```python
from build123d import *

# Parameters (mm, degrees)
SALIENTE_EXTRUIR1_DEPTH = 5
CORTAR_EXTRUIR1_DEPTH   = 15
SALIENTE_EXTRUIR2_DEPTH = 20
CORTAR_EXTRUIR2_DEPTH   = 30


with BuildPart() as part:
    # Croquis1 → Saliente-Extruir1 (new, symmetric)
    with BuildSketch(Plane.XY):
        Polygon((-2.5, 4), (2.5, -1), (-22.5, -8), (-22.5, -4), align=None)
        Polygon((22.5, 4), (-2.5, 4), (2.5, -1), (22.5, -1), align=None)
    extrude(amount=SALIENTE_EXTRUIR1_DEPTH, both=True)

    # Croquis3 → Cortar-Extruir1 (cut, symmetric)
    with BuildSketch(Plane(origin=(0, 0, 0), x_dir=(1, 0, 0), z_dir=(0, 1, 0))):
        Polygon((-22.5, 1.5), (-2.5, 5), (-22.5, 5), align=None)
        Polygon((-2.5, -5), (-22.5, -5), (-22.5, -1.5), align=None)
    extrude(amount=CORTAR_EXTRUIR1_DEPTH, both=True, mode=Mode.SUBTRACT)

    # Croquis5 → Saliente-Extruir2 (add)
    with BuildSketch(Plane.XY.offset(5)):
        Polygon((-2.5, 4), (-2.5, -2.4), (2.5, -1), (22.5, -1), (22.5, 4), align=None)
    extrude(amount=SALIENTE_EXTRUIR2_DEPTH)

    # Croquis2 → Cortar-Extruir2 (cut)
    with BuildSketch(Plane(origin=(0, 4, 0), x_dir=(1, 0, 0), z_dir=(0, 1, 0))):
        with BuildLine():
            Line((7.25, 0), (7.25, -20))
            ThreePointArc((7.25, -20), (6, -21.25), (4.75, -20))
            Line((4.75, -20), (4.75, 0))
            ThreePointArc((4.75, 0), (6, 1.25), (7.25, 0))
        make_face()
        with BuildLine():
            Line((15.25, 0), (15.25, -20))
            ThreePointArc((15.25, -20), (16.5, -21.25), (17.75, -20))
            Line((17.75, -20), (17.75, 0))
            ThreePointArc((17.75, 0), (16.5, 1.25), (15.25, 0))
        make_face()
    extrude(amount=-CORTAR_EXTRUIR2_DEPTH, mode=Mode.SUBTRACT)


solid = part.part
```
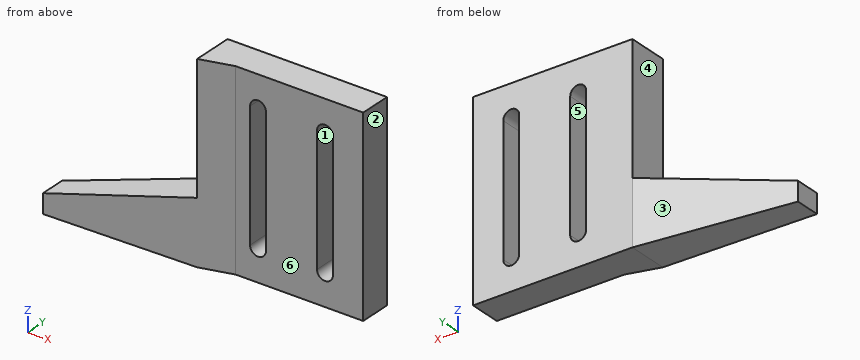
The listing builds one solid part. Answer for the finished solid, in the listing's coordinates (mm). Face numbers are marked on the shaded views. A direction names the side the tool comes from. Round coordinates to 2 decimals unless told otherwise and drop trailing zeros. Loops run counter-clockwise (first coordinate to the right, second up) from the corner with the lowest first, then second, coordinate; pieces in that order, holes last. Notation, with made-up numbers: (-20, 15) - (19, 15) arc R7 cw to (19, 28) - close; hole circle Ø2 at (53, 76.5). An arc over 180 degrees is marked (long way). Use one line per item in the form item = value. Start each with the question number.
1. A tool of negligible diameter and unlimited length cuts with its end or side. For the marked faces 4, 5 and 6, from which of +Z, -Z, +X, -X, +Y, -Y can it reach the whole face along a straight path? Write none if from no direction.
2. Consider line 1 (X direction, y = 0, z = 15.5); line 2 (Y direction, x = 8.5, z = 15); line 3 (X direction, y = 3.75, z = 22). Determine where each line is inside the solid, lowest interval first. Write a range as [from, to].
3. The part is cut by section D-D on z = 23. Determine the outline of the cut face in (x, y).
4. Given pin 1 Ø2 at (y, z) = (-0.5, 14.5) entering from -X; pin 2 Ø4 at (y, z) = (-5.5, 18) entering from +X; pin 3 Ø6 at (x, z) = (15, 14) entering from -Y; pin 4 Ø12 at (x, z) = (5.5, 20.5) entering from -Y, each flat-ended and moving along its own axis, determine where each tip first touches the part or whether it passes through.
5. The part is cut by section A-A on z = 12.5. Determine the outline of the cut face in (x, y).
6. The part is cut by section B-B on x = 6. Determine the outline of the cut face in (y, z).
7. For a pull along X with two mould halves and no side action, classify the marked faces 1, 2 and 3 as pulls with the +X half, pulls with the -X half, needs draft (parallel to the pull), parting line crosses it, or undercut.
8. The part is cut by section C-C on y = 2.25. Determine the outline of the cut face in (x, z) (3 decimals).
Geometry check:
q1.face_4 = +Z, -X, +Y, -Y
q1.face_5 = +Y, -Y
q1.face_6 = +Z, -Z, +X, -Y
q2.line_1 = [-2.5, 4.75], [7.25, 15.25], [17.75, 22.5]
q2.line_2 = [-1, 4]
q2.line_3 = [-2.5, 22.5]
q3.outline = (-2.5, -2.4) - (2.5, -1) - (22.5, -1) - (22.5, 4) - (-2.5, 4) - close
q4.pin_1 = -2.5
q4.pin_2 = through
q4.pin_3 = -1
q4.pin_4 = -1.84
q5.outline = (-2.5, -2.4) - (2.5, -1) - (4.75, -1) - (4.75, 4) - (-2.5, 4) - close; (7.25, -1) - (15.25, -1) - (15.25, 4) - (7.25, 4) - close; (17.75, -1) - (22.5, -1) - (22.5, 4) - (17.75, 4) - close
q6.outline = (-1, -5) - (4, -5) - (4, -1.25) - (-1, -1.25) - close; (-1, 21.25) - (4, 21.25) - (4, 25) - (-1, 25) - close
q7.face_1 = undercut
q7.face_2 = pulls with the +X half
q7.face_3 = pulls with the -X half
q8.outline = (-6.875, -4.234) - (-2.5, -5) - (22.5, -5) - (22.5, 25) - (-2.5, 25) - (-2.5, 5) - (-6.875, 4.234) - close; hole (4.75, 0) arc R1.25 ccw to (7.25, 0) - (7.25, 20) arc R1.25 ccw to (4.75, 20) - close; hole (15.25, 0) arc R1.25 ccw to (17.75, 0) - (17.75, 20) arc R1.25 ccw to (15.25, 20) - close
